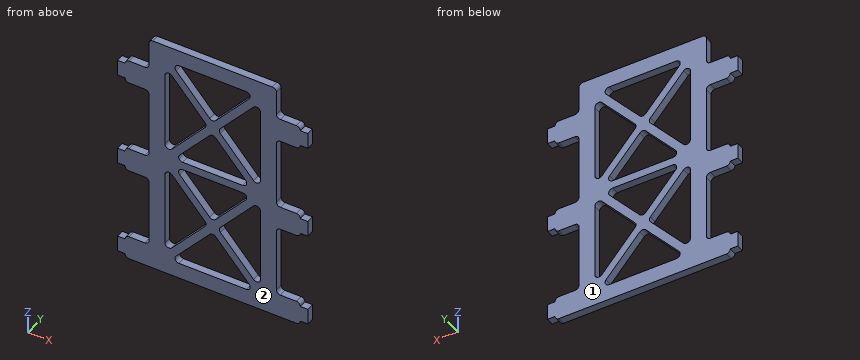
```python
from build123d import *

# Parameters (mm, degrees)
SKETCH1_W           = 50.8
SKETCH1_H           = 98.425
BOSS_EXTRUDE1_DEPTH = 1.5
SKETCH2_W           = 9.525
SKETCH2_H           = 9.525
BOSS_EXTRUDE2_DEPTH = 3
CUT_EXTRUDE1_DEPTH  = 3
FILLET1_R           = 1.5875
SKETCH5_W           = 3
SKETCH5_H           = 6.35
BOSS_EXTRUDE3_DEPTH = 3


with BuildPart() as part:
    # Sketch1 → Boss-Extrude1 (new, symmetric)
    with BuildSketch(Plane(origin=(0, 34.29, 0), x_dir=(1, 0, 0), z_dir=(0, 1, 0))):
        with Locations((0, 120.65)):
            Rectangle(SKETCH1_W, SKETCH1_H)
    extrude(amount=BOSS_EXTRUDE1_DEPTH, both=True)

    # Sketch2 → Boss-Extrude2 (add)
    with BuildSketch(Plane(origin=(0, 35.79, 0), x_dir=(1, 0, 0), z_dir=(0, 1, 0))):
        with Locations((30.1625, 165.1)):
            Rectangle(SKETCH2_W, SKETCH2_H)
        with Locations((-30.1625, 165.1)):
            Rectangle(SKETCH2_W, SKETCH2_H)
        with Locations((30.1625, 127)):
            Rectangle(SKETCH2_W, SKETCH2_H)
        with Locations((-30.1625, 127)):
            Rectangle(SKETCH2_W, SKETCH2_H)
        with Locations((30.1625, 88.9)):
            Rectangle(SKETCH2_W, SKETCH2_H)
        with Locations((-30.1625, 88.9)):
            Rectangle(SKETCH2_W, SKETCH2_H)
    extrude(amount=-BOSS_EXTRUDE2_DEPTH)

    # Sketch4 → Cut-Extrude1 (cut)
    with BuildSketch(Plane(origin=(0, 35.79, 0), x_dir=(1, 0, 0), z_dir=(0, 1, 0))):
        Polygon((16.925996512, 163.5125), (-16.925996512, 163.5125), (0, 144.470753924), align=None)
        Polygon((-2.124003488, 142.08125), (-19.05, 161.122996076), (-19.05, 123.039503924), align=None)
        Polygon((19.05, 161.122996076), (2.124003488, 142.08125), (19.05, 123.039503924), align=None)
        Polygon((15.514885401, 122.2375), (0, 139.691746076), (-15.514885401, 122.2375), align=None)
        Polygon((-2.124003488, 99.21875), (-19.05, 118.260496076), (-19.05, 80.177003924), align=None)
        Polygon((15.514885401, 119.0625), (-15.514885401, 119.0625), (0, 101.608253924), align=None)
        Polygon((19.05, 80.177003924), (19.05, 118.260496076), (2.124003488, 99.21875), align=None)
        Polygon((16.925996512, 77.7875), (0, 96.829246076), (-16.925996512, 77.7875), align=None)
    extrude(amount=-CUT_EXTRUDE1_DEPTH, mode=Mode.SUBTRACT)

    # Fillet1
    fillet1_edges = [part.edges().sort_by_distance(p)[0] for p in [
        (15.514885401, 34.29, -122.2375),
        (-15.514885401, 34.29, -122.2375),
        (0, 34.29, -139.691746076),
        (15.514885401, 34.29, -119.0625),
        (0, 34.29, -101.608253924),
        (-15.514885401, 34.29, -119.0625),
        (16.925996512, 34.29, -77.7875),
        (-16.925996512, 34.29, -77.7875),
        (0, 34.29, -96.829246076),
        (-2.124003488, 34.29, -99.21875),
        (-19.05, 34.29, -80.177003924),
        (-19.05, 34.29, -118.260496076),
        (-2.124003488, 34.29, -142.08125),
        (-19.05, 34.29, -123.039503924),
        (-19.05, 34.29, -161.122996076),
        (19.05, 34.29, -123.039503924),
        (2.124003488, 34.29, -142.08125),
        (19.05, 34.29, -161.122996076),
        (0, 34.29, -144.470753924),
        (-16.925996512, 34.29, -163.5125),
        (16.925996512, 34.29, -163.5125),
        (19.05, 34.29, -118.260496076),
        (19.05, 34.29, -80.177003924),
        (2.124003488, 34.29, -99.21875),
        (34.925, 34.29, -84.1375),
        (34.925, 34.29, -93.6625),
        (25.4, 34.29, -93.6625),
        (25.4, 34.29, -84.1375),
        (-25.4, 34.29, -122.2375),
        (-25.4, 34.29, -131.7625),
        (-34.925, 34.29, -131.7625),
        (-34.925, 34.29, -122.2375),
        (34.925, 34.29, -122.2375),
        (34.925, 34.29, -131.7625),
        (25.4, 34.29, -131.7625),
        (25.4, 34.29, -122.2375),
        (-25.4, 34.29, -160.3375),
        (-34.925, 34.29, -169.8625),
        (-34.925, 34.29, -160.3375),
        (-25.4, 34.29, -84.1375),
        (-25.4, 34.29, -93.6625),
        (-34.925, 34.29, -93.6625),
        (-34.925, 34.29, -84.1375),
        (34.925, 34.29, -160.3375),
        (34.925, 34.29, -169.8625),
        (25.4, 34.29, -160.3375),
        (-25.4, 34.29, -71.4375),
        (25.4, 34.29, -71.4375),
    ]]
    fillet(fillet1_edges, radius=FILLET1_R)

    # Sketch5 → Boss-Extrude3 (add)
    with BuildSketch(Plane(origin=(0, 35.79, 0), x_dir=(1, 0, 0), z_dir=(0, 1, 0))):
        with Locations((36.425, 165.1)):
            Rectangle(SKETCH5_W, SKETCH5_H)
        with Locations((-36.425, 165.1)):
            Rectangle(SKETCH5_W, SKETCH5_H)
        with Locations((36.425, 127)):
            Rectangle(SKETCH5_W, SKETCH5_H)
        with Locations((-36.425, 127)):
            Rectangle(SKETCH5_W, SKETCH5_H)
        with Locations((36.425, 88.9)):
            Rectangle(SKETCH5_W, SKETCH5_H)
        with Locations((-36.425, 88.9)):
            Rectangle(SKETCH5_W, SKETCH5_H)
    extrude(amount=-BOSS_EXTRUDE3_DEPTH)


solid = part.part
```
Here's how the part is built. I have some questions about the finished solid (model axes, mm). Face numbers are marked on the shaded views. Coordinates: 2 decimals unless noted, no trailing zeros. Loops run counter-clockwise (first coordinate to the right, second up) from the corner with the lowest first, then second, coordinate; pieces in that order, holes last. Notation, with made-up numbers: (40, 51.25) -> (47, 51.25) arc R12 ccw to (47, 59.25) -> close; hole circle Ø2 at (20, 57.5). An arc over 180 degrees is marked (long way). Return JSON: item names as keys, results as strings.
1) I need wall thicknesses on line 1 (Z direction, x = -30, y = 34.1); line 2 (X direction, y = 35.25, z = -100.5); line 3 (X direction, y = 33.55, z = -132.5). Which ranges of each line are inside material? Lowest first, please. Write a range as from..to.
Results below:
{"line 1": "-169.86..-160.34, -131.76..-122.24, -93.66..-84.14", "line 2": "-25.4..-19.05, -3.26..3.26, 19.05..25.4", "line 3": "-25.65..-19.05, -10.64..-6.39, 6.39..10.64, 19.05..25.65"}
2) If we section it at A-A, the plane z = -106: Write out the boundary of the cut face in (x, y).
Results below:
{"outline": "(-25.4, 32.79) -> (-19.05, 32.79) -> (-19.05, 35.79) -> (-25.4, 35.79) -> close; (-8.15, 32.79) -> (-3.9, 32.79) -> (-3.9, 35.79) -> (-8.15, 35.79) -> close; (3.9, 32.79) -> (8.15, 32.79) -> (8.15, 35.79) -> (3.9, 35.79) -> close; (19.05, 32.79) -> (25.4, 32.79) -> (25.4, 35.79) -> (19.05, 35.79) -> close"}
3) If we section it at D-D, the plane y = 34.75: Count the separate pieces of the cut face and the enclosed holes in it, then the cut area to 3 significant figures.
Results below:
{"separate pieces": "1", "enclosed holes": "8", "area": "3,240 mm²"}
4) If we section it at C-C, the plane x = -5: Write out the boundary of the cut face in (y, z), then the cut area to 3 significant figures.
Results below:
{"outline": "(32.79, -169.86) -> (35.79, -169.86) -> (35.79, -163.51) -> (32.79, -163.51) -> close; (32.79, -150.1) -> (35.79, -150.1) -> (35.79, -145.32) -> (32.79, -145.32) -> close; (32.79, -138.85) -> (35.79, -138.85) -> (35.79, -134.07) -> (32.79, -134.07) -> close; (32.79, -122.24) -> (35.79, -122.24) -> (35.79, -119.06) -> (32.79, -119.06) -> close; (32.79, -107.23) -> (35.79, -107.23) -> (35.79, -102.45) -> (32.79, -102.45) -> close; (32.79, -95.98) -> (35.79, -95.98) -> (35.79, -91.2) -> (32.79, -91.2) -> close; (32.79, -77.79) -> (35.79, -77.79) -> (35.79, -71.44) -> (32.79, -71.44) -> close", "area": "105 mm²"}
5) Thinking about a two-plate mould opening in Y: for the marked faces 1 and 2, which applies, +Y half, -Y half, draft (parallel to the pull), parting line (faces both ways), or undercut?
Results below:
{"face 1": "+Y half", "face 2": "-Y half"}
6) If we section it at B-B, the plane z = -79: Write out the boundary of the cut face in (x, y), then the cut area to 3 significant figures.
Results below:
{"outline": "(-25.4, 32.79) -> (-14.93, 32.79) -> (-14.93, 35.79) -> (-25.4, 35.79) -> close; (14.93, 32.79) -> (25.4, 32.79) -> (25.4, 35.79) -> (14.93, 35.79) -> close", "area": "62.8 mm²"}
7) Will these pins go through, and if not, where does the flat tip stop? pin 1 (0.9 mm diameter, centred on x = 31, y = 35, fed in from +Z); pin 2 (1.5 mm diameter, centred on x = -36, y = 34.5, fed in from +Z) (3 decimals).
Results below:
{"pin 1": "z = -84.14", "pin 2": "z = -85.725"}
